from build123d import *

# Parameters (mm, degrees)
SKETCH1_W                  = 150
SKETCH1_H                  = 55
MAINPCB_DEPTH              = 1.6
SKETCH2_R                  = 1.5
SCREWHOLES_DEPTH           = 80.898748426
SKETCH3_W                  = 98.5
SKETCH3_H                  = 60
BOSS_EXTRUDE2_DEPTH        = 4.2
SKETCH4_W                  = 97
SKETCH4_H                  = 40
BOSS_EXTRUDE3_DEPTH        = 9.5
SKETCH5_R                  = 6
SKETCH5_W                  = 13
SKETCH5_H                  = 13
SKETCH5_W_2                = 6
SKETCH5_H_2                = 6
BOSS_EXTRUDE4_DEPTH        = 4.4
SKETCH6_R                  = 1.5
BOSS_EXTRUDE5_DEPTH        = 2
SKETCH7_R                  = 6
BOSS_EXTRUDE6_DEPTH        = 7
SKETCH8_R                  = 3.5
BOSS_EXTRUDE7_DEPTH        = 9.3
SKETCH9_R                  = 7.5
BOSS_EXTRUDE8_DEPTH        = 15
BOSS_EXTRUDE8_TAPER        = 6
SKETCH10_W                 = 40
SKETCH10_H                 = 1.5
ANNOYINGLYPLACEDPINS_DEPTH = 5


with BuildPart() as part:
    # Sketch1 → MainPCB (new body)
    with BuildSketch(Plane(origin=(0, 0, 0), x_dir=(1, 0, 0), z_dir=(0, 1, 0))):
        Rectangle(SKETCH1_W, SKETCH1_H)
    extrude(amount=MAINPCB_DEPTH)

    # Sketch2 → ScrewHoles (cut, through all)
    with BuildSketch(Plane(origin=(0, 1.6, 0), x_dir=(1, 0, 0), z_dir=(0, 1, 0))):
        with Locations(Location((-72.5, 24.75, 0), (0, 0, 270))):
            Circle(SKETCH2_R)
        with Locations(Location((-72.5, -24.75, 0), (0, 0, 90))):
            Circle(SKETCH2_R)
        with Locations(Location((72.5, -24.75, 0), (0, 0, 270))):
            Circle(SKETCH2_R)
        with Locations(Location((72.5, 24.75, 0), (0, 0, 90))):
            Circle(SKETCH2_R)
    extrude(amount=-SCREWHOLES_DEPTH, mode=Mode.SUBTRACT)

    # Sketch3 → Boss-Extrude2 (add)
    with BuildSketch(Plane(origin=(0, 1.6, 0), x_dir=(1, 0, 0), z_dir=(0, 1, 0))):
        with Locations((-11.75, -4.5)):
            Rectangle(SKETCH3_W, SKETCH3_H)
    extrude(amount=BOSS_EXTRUDE2_DEPTH)

    # Sketch4 → Boss-Extrude3 (add)
    with BuildSketch(Plane(origin=(0, 5.8, 0), x_dir=(1, 0, 0), z_dir=(0, 1, 0))):
        with Locations((-12, -5.5)):
            Rectangle(SKETCH4_W, SKETCH4_H)
    extrude(amount=BOSS_EXTRUDE3_DEPTH)

    # Sketch5 → Boss-Extrude4 (add)
    with BuildSketch(Plane(origin=(0, 1.6, 0), x_dir=(1, 0, 0), z_dir=(0, 1, 0))):
        with Locations(Location((62.5, 16.5, 0), (0, 0, 90))):
            Circle(SKETCH5_R)
        with Locations((62.5, -2.45)):
            Rectangle(SKETCH5_W, SKETCH5_H)
        with Locations((62.5, -20.15)):
            Rectangle(SKETCH5_W_2, SKETCH5_H_2)
    extrude(amount=BOSS_EXTRUDE4_DEPTH)

    # Sketch6 → Boss-Extrude5 (add)
    with BuildSketch(Plane(origin=(0, 6, 0), x_dir=(1, 0, 0), z_dir=(0, 1, 0))):
        with Locations(Location((62.5, -20.15, 0), (0, 0, 270))):
            Circle(SKETCH6_R)
    extrude(amount=BOSS_EXTRUDE5_DEPTH)

    # Sketch7 → Boss-Extrude6 (add)
    with BuildSketch(Plane(origin=(0, 6, 0), x_dir=(1, 0, 0), z_dir=(0, 1, 0))):
        with Locations(Location((62.5, 16.5, 0), (0, 0, 90))):
            Circle(SKETCH7_R)
    extrude(amount=BOSS_EXTRUDE6_DEPTH)

    # Sketch8 → Boss-Extrude7 (add)
    with BuildSketch(Plane(origin=(0, 6, 0), x_dir=(1, 0, 0), z_dir=(0, 1, 0))):
        with Locations(Location((62.5, -2.45, 0), (0, 0, 90))):
            Circle(SKETCH8_R)
    extrude(amount=BOSS_EXTRUDE7_DEPTH)

    # Sketch9 → Boss-Extrude8 (add)
    with BuildSketch(Plane(origin=(0, 15.3, 0), x_dir=(1, 0, 0), z_dir=(0, 1, 0))):
        with Locations((62.5, -2.45)):
            Circle(SKETCH9_R)
    extrude(amount=BOSS_EXTRUDE8_DEPTH, taper=BOSS_EXTRUDE8_TAPER)

    # Sketch10 → AnnoyinglyPlacedPins (add)
    with BuildSketch(Plane(origin=(0, 5.8, 0), x_dir=(1, 0, 0), z_dir=(0, 1, 0))):
        with Locations((-32, 21.75)):
            Rectangle(SKETCH10_W, SKETCH10_H)
    extrude(amount=ANNOYINGLYPLACEDPINS_DEPTH)


solid = part.part
The listing builds one solid part. Answer for the finished solid, in the listing's coordinates (mm). A direction names the side the tool comes from. Give positions to 0.01 mm unless a question says otherwise; leave off trailing zeros. Loops run counter-clockwise (first coordinate to the right, second up) from the corner with the lowest first, then second, coordinate; pieces in that order, holes last.
Item 1: A cutting plane is placed at C-C (x = 25). Give the vertices of the cut face in (y, z), then the cut area to 3 significant figures.
Derived:
outline: (0, -27.5) - (1.6, -27.5) - (1.6, -25.5) - (5.8, -25.5) - (5.8, -14.5) - (15.3, -14.5) - (15.3, 25.5) - (5.8, 25.5) - (5.8, 34.5) - (1.6, 34.5) - (1.6, 27.5) - (0, 27.5) - close
area: 720 mm2
Item 2: A cutting plane is placed at D-D (z = 20). Give the vertices of the cut face in (x, y), then the cut area to 3 significant figures.
Derived:
outline: (-75, 0) - (75, 0) - (75, 1.6) - (65.5, 1.6) - (65.5, 6) - (63.99, 6) - (63.99, 8) - (61.01, 8) - (61.01, 6) - (59.5, 6) - (59.5, 1.6) - (37.5, 1.6) - (37.5, 5.8) - (36.5, 5.8) - (36.5, 15.3) - (-60.5, 15.3) - (-60.5, 5.8) - (-61, 5.8) - (-61, 1.6) - (-75, 1.6) - close
area: 1,610 mm2
Item 3: A tool of negligible diameter and unlimited length cuts with its end or side. For faces 4 (the flat face through (64, 15.3, 6)), 5 (the flat face through (62, 13, -16)), 6 (the flat face through (36.5, 10, 6)), 7 (the flat face through (-12, 1.6, 31)), from which of +Z, -Z, +X, -X, +Y, -Y can it reach the whole face along a straight path? Write none if from no direction.
Derived:
face 4: none
face 5: -Z, +X, +Y
face 6: +Z, -Z, +Y
face 7: +Z, +X, -X, -Y
Item 4: Determine the mould class of faces 1 (the flat face through (56, 4, 3)), 2 (the flat face through (65.5, 4, 20)), 3 (the flat face through (62, 30.3, 2)) for opening direction X: +X half, -X half, draft (parallel to the pull), parting line (faces both ways), or undercut.
Derived:
face 1: undercut
face 2: +X half
face 3: draft
Item 5: A cutting plane is placed at B-B (z = -16.5). Give the vertices of the cut face in (x, y), then the cut area to 4 significant figures.
Derived:
outline: (-75, 0) - (75, 0) - (75, 1.6) - (68.5, 1.6) - (68.5, 13) - (56.5, 13) - (56.5, 1.6) - (37.5, 1.6) - (37.5, 5.8) - (-61, 5.8) - (-61, 1.6) - (-75, 1.6) - close
area: 790.5 mm2
Item 6: Find the intervals of material crossed by line 1 along Z through (x, y) = (72.5, 0.75); line 2 along X through (y, z) = (0.6, 24.75); line 3 along X through (y, z) = (4, 19), in increasing order.
Derived:
line 1: z = -27.5 to -26.25, -23.25 to 23.25, 26.25 to 27.5
line 2: x = -75 to -74, -71 to 71, 74 to 75
line 3: x = -61 to 37.5, 59.5 to 65.5
Item 7: A cutting plane is placed at A-A (x = -72.5). Give the vertices of the cut face in (y, z).
Derived:
outline: (0, -27.5) - (1.6, -27.5) - (1.6, -26.25) - (0, -26.25) - close; (0, -23.25) - (1.6, -23.25) - (1.6, 23.25) - (0, 23.25) - close; (0, 26.25) - (1.6, 26.25) - (1.6, 27.5) - (0, 27.5) - close
Item 8: Each of these flat-tipped pins is pushed along its axis until it touches: pin 1 Ø10.5 at (y, z) = (9, 10) entering from -X; pin 2 Ø8 at (x, z) = (-56, 13) entering from +Y; pin 3 Ø5 at (x, y) = (62, 4.5) entering from -Z. Where does it stop, or does it pass through?
Derived:
pin 1: stops at x = -61
pin 2: stops at y = 15.3
pin 3: stops at z = -22.5
